from build123d import *

# Parameters (mm, degrees)
SKETCH1_R           = 4
BOSS_EXTRUDE1_DEPTH = 1.5


with BuildPart() as part:
    # Sketch1 → Boss-Extrude1 (new, symmetric)
    with BuildSketch(Plane(origin=(0, 0, 0), x_dir=(1, 0, 0), z_dir=(0, 1, 0))):
        with BuildLine():
            Line((5.562177826, 3.788675135), (0.5, 6.711324865))
            ThreePointArc((0.5, 6.711324865), (0, 6.845299462), (-0.5, 6.711324865))
            Line((-0.5, 6.711324865), (-5.562177826, 3.788675135))
            ThreePointArc((-5.562177826, 3.788675135), (-5.92820323, 3.422649731), (-6.062177826, 2.922649731))
            Line((-6.062177826, 2.922649731), (-6.062177826, -2.922649731))
            ThreePointArc((-6.062177826, -2.922649731), (-5.92820323, -3.422649731), (-5.562177826, -3.788675135))
            Line((-5.562177826, -3.788675135), (-0.5, -6.711324865))
            ThreePointArc((-0.5, -6.711324865), (0, -6.845299462), (0.5, -6.711324865))
            Line((0.5, -6.711324865), (5.562177826, -3.788675135))
            ThreePointArc((5.562177826, -3.788675135), (5.92820323, -3.422649731), (6.062177826, -2.922649731))
            Line((6.062177826, -2.922649731), (6.062177826, 2.922649731))
            ThreePointArc((6.062177826, 2.922649731), (5.92820323, 3.422649731), (5.562177826, 3.788675135))
        make_face()
        with Locations(Location((0, 0, 0), (0, 0, 270))):
            Circle(SKETCH1_R, mode=Mode.SUBTRACT)
    extrude(amount=BOSS_EXTRUDE1_DEPTH, both=True)


solid = part.part
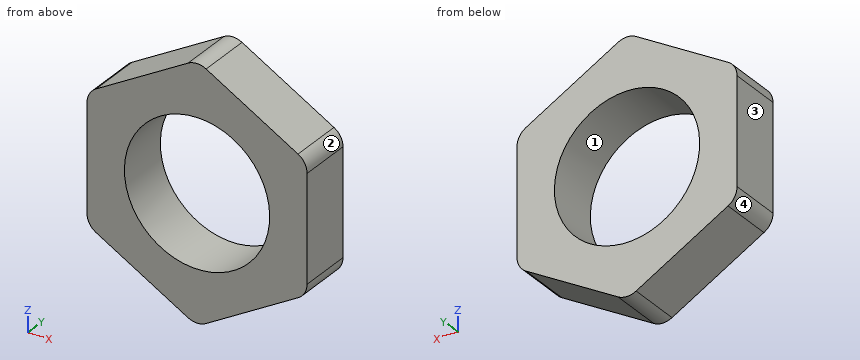
Geometry: final body of the model. Coordinates: model frame, mm. Face numbers are marked on the shaded views. Give positions to 0.01 mm unless a question says otherwise; leave off trailing zeros. Loops run counter-clockwise (first coordinate to the right, second up) from the corner with the lowest first, then second, coordinate; pieces in that order, holes last. Notation, with made-up numbers: M 57.25,-6 L 97.25,-6 A18 ccw 97.25,-2 Z; hole C 60,88.25 d3. An arc over 180 degrees is marked long. Put each result on its own line as item: value. Start each with the question number.
1) Cut plane B-B (z = 0). Output: boundary loops of the cut face in (x, y), then the cut area to 3 significant figures.
2) Cut plane C-C (y = 1.1). Output: boundary loops of the cut face in (x, z).
3) Contact query for flat-ended pins moving along their axis: pin 1 (5 mm diameter, centred on x = 0, z = 0, fed in from +Y); pin 2 (1.5 mm diameter, centred on x = 3.5, y = 0.5, fed in from +Z). Output: stop coordinate, or through.
4) Cut plane A-A (x = 0). Output: boundary loops of the cut face in (y, z).
5) Cut plane D-D (z = -5). Output: boundary loops of the cut face in (x, y).
6) Pull-direction query (Z, two-part tool) for the marked faces 1, 2, 3 and 4; classes: pulls with the +Z half, pulls with the -Z half, needs draft (parallel to the pull), parting line crosses it, or undercut.
7) Ray query, line 1 along X through (y, z) = (0.35, 0); line 2 along X through (y, z) = (-0.4, -0.75); line 3 along Z through (x, y) = (1.5, -0.9). Return the intervals inside material, ascending.
Verdict:
1. outline: M -6.06,-1.5 L -4,-1.5 L -4,1.5 L -6.06,1.5 Z; M 4,-1.5 L 6.06,-1.5 L 6.06,1.5 L 4,1.5 Z
1. area: 12.4 mm2
2. outline: M -6.06,-2.92 A1 ccw -5.56,-3.79 L -0.5,-6.71 A1 ccw 0.5,-6.71 L 5.56,-3.79 A1 ccw 6.06,-2.92 L 6.06,2.92 A1 ccw 5.56,3.79 L 0.5,6.71 A1 ccw -0.5,6.71 L -5.56,3.79 A1 ccw -6.06,2.92 Z; hole C 0,0 d8
3. pin 1: through
3. pin 2: z = 5.41
4. outline: M -1.5,-6.85 L 1.5,-6.85 L 1.5,-4 L -1.5,-4 Z; M -1.5,4 L 1.5,4 L 1.5,6.85 L -1.5,6.85 Z
5. outline: M -3.46,-1.5 L 3.46,-1.5 L 3.46,1.5 L -3.46,1.5 Z
6. face 1: undercut
6. face 2: pulls with the +Z half
6. face 3: needs draft
6. face 4: pulls with the -Z half
7. line 1: -6.06 to -4, 4 to 6.06
7. line 2: -6.06 to -3.93, 3.93 to 6.06
7. line 3: -6.13 to -3.71, 3.71 to 6.13
